Read the model definition and answer for the solid it produces. Units are mm, in the model's axes. A direction names the side the tool comes from. Coordinates: 2 decimals unless noted, no trailing zeros. Write each loop counter-clockwise with the first axis right and the second up, starting at its lowest first coordinate (ties: lowest second). Pieces come first, ordered by that corner, then holes.
Item 1: Determine the mould class of faces 3 (the face through (29.62, 14, 3)), 4 (the face through (39, 14, 0)), 5 (the face through (23.432, 14, 3)), 6 (the face through (58.024, 13.945, 2.958)) for opening direction Y: released by +Y, released by -Y, zero draft, split by the parting line, or undercut.
Item 2: Section D-D (y = 20.75) is taken. Give the vertices of the cut face in (x, z).
Item 3: Each of these flat-tipped pins is pushed along its axis until it touches: P1, Ø3, axis at y = 9, z = 4.5, coming from the -X side; P2, Ø2, axis at x = 51.5, z = 0.5, coming from the -Y side. Where does it stop, or does it pass through?
Item 4: Section A-A (y = 15.25) is taken. Give the vertices of the cut face in (x, z).
Item 5: Straight lines are drawn through the part: probe 1 along Y at (x, z) = (26.5, 1.95); probe 2 along X at (y, z) = (12.75, 0.65); probe 3 along X at (y, z) = (15, 3.9). For each, find the intervals that lie inside material, in ascending order.
Item 6: Section B-B (z = 5.4) is taken. Give the vertices of the cut face in (x, y).
Item 7: A tool of negligible diameter and unlimited length cuts with its end or side. For faces 1 (the face through (26, 10.675, 3)), 2 (the face through (18.53, 13.59, 2.96)), from which of +Z, -Z, +X, -X, +Y, -Y can it reach the whole face along a straight path? Write none if from no direction.
Item 8: Section C-C (x = 25) is taken. Give the vertices of the cut face in (y, z).
from build123d import *

# Parameters (mm, degrees)
MODEL_R             = 2
BOSS_EXTRUDE1_DEPTH = 6


with BuildPart() as part:
    # Model → Boss-Extrude1 (new body)
    with BuildSketch(Plane.XY):
        with BuildLine():
            Line((26.526195336, 21.768592837), (50.026195336, 21.768592837))
            ThreePointArc((50.026195336, 21.768592837), (58.026195336, 13.768592837), (50.026195336, 5.768592837))
            Line((50.026195336, 5.768592837), (26.526195336, 5.768592837))
            ThreePointArc((26.526195336, 5.768592837), (18.526195336, 13.768592837), (26.526195336, 21.768592837))
        make_face()
        with Locations((50.026195336, 13.768592837)):
            Circle(MODEL_R, mode=Mode.SUBTRACT)
        Polygon((29.619945336, 13.768592837), (29.619945336, 16.862342837), (23.432445336, 16.862342837), (23.432445336, 10.674842837), (29.619945336, 10.674842837), align=None, mode=Mode.SUBTRACT)
    extrude(amount=BOSS_EXTRUDE1_DEPTH)


solid = part.part
Established:
1. face 3: undercut
1. face 4: zero draft
1. face 5: undercut
1. face 6: split by the parting line
2. outline: (22.62, 0) - (53.93, 0) - (53.93, 6) - (22.62, 6) - close
3. P1: stops at x = 19.22
3. P2: stops at y = 5.78
4. outline: (18.66, 0) - (23.43, 0) - (23.43, 6) - (18.66, 6) - close; (29.62, 0) - (48.68, 0) - (48.68, 6) - (29.62, 6) - close; (51.37, 0) - (57.89, 0) - (57.89, 6) - (51.37, 6) - close
5. probe 1: y = 5.77 to 10.67, 16.86 to 21.77
5. probe 2: x = 18.59 to 23.43, 29.62 to 48.31, 51.75 to 57.96
5. probe 3: x = 18.62 to 23.43, 29.62 to 48.45, 51.6 to 57.93
6. outline: (26.53, 5.77) - (50.03, 5.77) arc R8 ccw to (50.03, 21.77) - (26.53, 21.77) arc R8 ccw to start; hole (23.43, 10.67) - (29.62, 10.67) - (29.62, 16.86) - (23.43, 16.86) - close; hole circle Ø4 at (50.03, 13.77)
7. face 1: +Z, -Z
7. face 2: +Z, -Z, -X
8. outline: (5.92, 0) - (10.67, 0) - (10.67, 6) - (5.92, 6) - close; (16.86, 0) - (21.62, 0) - (21.62, 6) - (16.86, 6) - close
